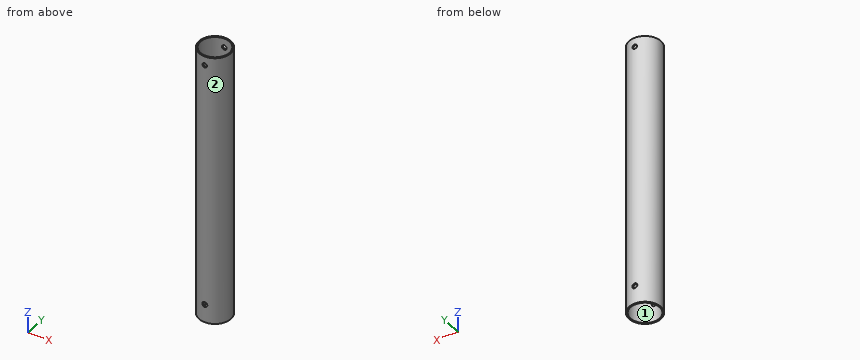
```python
from build123d import *

# Parameters (mm, degrees)
SKETCH1_R               = 17.5
SKETCH1_R_2             = 15.9125
BOSS_EXTRUDE1_DEPTH     = 150
SKETCH5_W               = 2.75
SKETCH5_H               = 17.5
SKETCH6_R               = 2.5
CUT_EXTRUDE1_DEPTH      = 18.5000001
CUT_EXTRUDE1_DEPTH_BACK = 18.5000001


with BuildPart() as part:
    # Sketch1 → Boss-Extrude1 (new body, symmetric)
    with BuildSketch(Plane.XY):
        Circle(SKETCH1_R)
        Circle(SKETCH1_R_2, mode=Mode.SUBTRACT)
    extrude(amount=BOSS_EXTRUDE1_DEPTH, both=True)

    # Sketch5 → M5 Clearance Hole1 (revolve, cut)
    with BuildSketch(Plane(origin=(0, 0, -130), x_dir=(0, 0, -1), z_dir=(1, 0, 0))):
        with Locations((1.375, 8.75)):
            Rectangle(SKETCH5_W, SKETCH5_H)
    m5_clearance_hole1 = revolve(axis=Axis((0, -6.35, -130), (0, 1, 0)), mode=Mode.SUBTRACT)

    # Mirror1: M5 Clearance Hole1 across plane
    add(m5_clearance_hole1.mirror(Plane.ZX), mode=Mode.SUBTRACT)

    # Sketch6 → Cut-Extrude1 (cut, two sides)
    with BuildSketch(Plane(origin=(0, 0, 0), x_dir=(1, 0, 0), z_dir=(0, 1, 0))) as cut_extrude1_sk:
        with Locations((0, -140)):
            Circle(SKETCH6_R)
    extrude(amount=CUT_EXTRUDE1_DEPTH, mode=Mode.SUBTRACT)
    extrude(cut_extrude1_sk.sketch, amount=-CUT_EXTRUDE1_DEPTH_BACK, mode=Mode.SUBTRACT)


solid = part.part
```
Check sheet for the modelled part. Datum: model origin and axes. Units: mm. Face numbers are marked on the shaded views. Give positions to 0.01 mm unless a question says otherwise; leave off trailing zeros. Write each loop counter-clockwise with the first axis right and the second up, starting at its lowest first coordinate (ties: lowest second). Pieces come first, ordered by that corner, then holes. Notation, with made-up numbers: (38.25, -8.5) - (51.25, -8.5) arc R21 cw to (51.25, 30.5) - close; hole circle Ø11 at (45.25, -39). An arc over 180 degrees is marked (long way). Answer as a JSON object with one key per item and string values. Group by question number.
1) Sectioned sample at B-B (y = -4). Record the cut outline in (x, z).
2) Sectioned sample at D-D (z = -47). Record the cut outline in (x, y) (1 decimal).
3) Release check for a two-part mould opening along Y. For the marked faces 1 and 2 record: pulls with the +Y half, pulls with the -Y half, needs draft (parallel to the pull), parting line crosses it, or undercut.
4) Depth check by flat-ended pin: P1, Ø2, axis at x = 9.5, z = 7, coming from the +Y side; P2, Ø5, axis at x = 0, z = -130, coming from the +Y side; P3, Ø6, axis at x = 8, z = -87, coming from the +Y side; P4, Ø12, axis at y = -12, z = -22.5, coming from the -X side. Enter the tip coordinate at first touch or a pass-through.
5) Sectioned sample at A-A (x = 0). Record the cut outline in (y, z).
6) Thickness scan on probe 1 along Z at (x, y) = (0, 16); probe 2 along Y at (x, z) = (1, -87.5); probe 3 along Y at (x, z) = (-9, -121). Record the ranges inside material, lowest first. Write a range as from..to.
Geometry results:
{
 "1": {"outline": "(-17.04, -150) - (-15.4, -150) - (-15.4, 150) - (-17.04, 150) - close; (15.4, -150) - (17.04, -150) - (17.04, 150) - (15.4, 150) - close"},
 "2": {"outline": "circle Ø35 at (0, 0); hole circle Ø31.8 at (0, 0)"},
 "3": {"face 1": "undercut", "face 2": "parting line crosses it"},
 "4": {"P1": "stops at y = 15.3", "P2": "passes through", "P3": "stops at y = 16.77", "P4": "stops at x = -16.44"},
 "5": {"outline": "(-17.5, -150) - (-15.91, -150) - (-15.91, -132.75) - (-17.5, -132.75) - close; (-17.5, -127.25) - (-15.91, -127.25) - (-15.91, 137.5) - (-17.5, 137.5) - close; (-17.5, 142.5) - (-15.91, 142.5) - (-15.91, 150) - (-17.5, 150) - close; (15.91, -150) - (17.5, -150) - (17.5, -132.75) - (15.91, -132.75) - close; (15.91, -127.25) - (17.5, -127.25) - (17.5, 137.5) - (15.91, 137.5) - close; (15.91, 142.5) - (17.5, 142.5) - (17.5, 150) - (15.91, 150) - close"},
 "6": {"probe 1": "z = -150..-132.75, -127.25..137.5, 142.5..150", "probe 2": "y = -17.47..-15.88, 15.88..17.47", "probe 3": "y = -15.01..-13.12, 13.12..15.01"}
}
